Check sheet for the drawn part. Datum: minimum x, y, z corner. Units: mm. Coordinates: 2 decimals unless noted, no trailing zeros. Loops run counter-clockwise (first coordinate to the right, second up) from the corner with the lowest first, then second, coordinate; pieces in that order, holes last.
Q1. Material ranges on probe 1 along X at (y, z) = (16.5, 1.2); probe 2 along Y at (x, z) = (29, 1.2), recorded low to high.
Q2. Sectioned sample at A-A (y = 13.25). Enter the section's corners in (x, z), then the cut area to 3 significant figures.
Q3. Sectioned sample at B-B (z = 0.7). Enter the section's corners in (x, y).
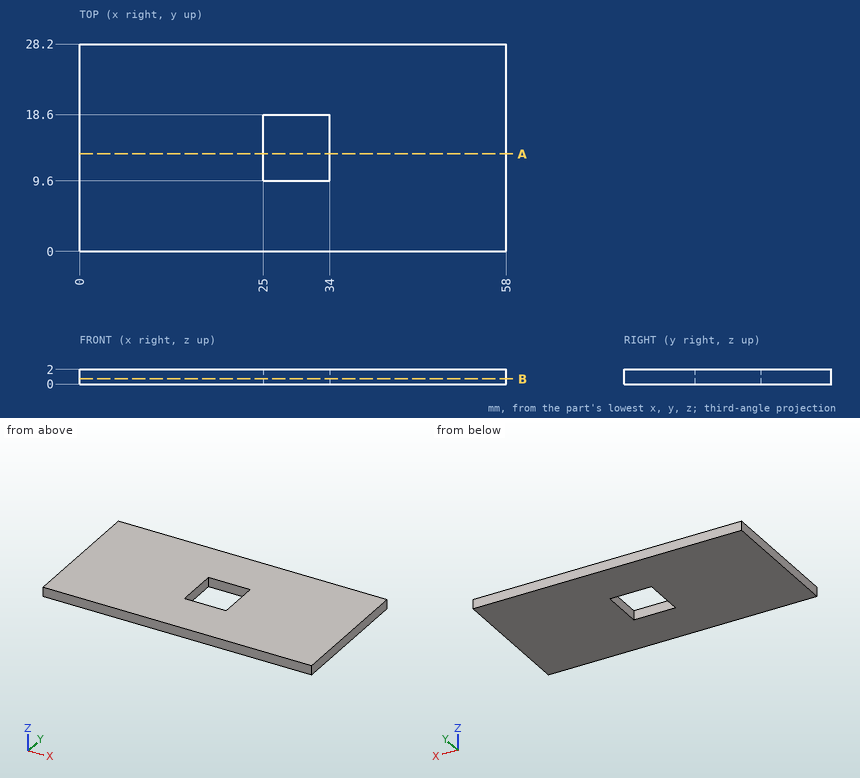
Geometry check:
1. probe 1: x = 0 to 25, 34 to 58
1. probe 2: y = 0 to 9.6, 18.6 to 28.2
2. outline: (0, 0) - (25, 0) - (25, 2) - (0, 2) - close; (34, 0) - (58, 0) - (58, 2) - (34, 2) - close
2. area: 98.0 mm2
3. outline: (0, 0) - (58, 0) - (58, 28.2) - (0, 28.2) - close; hole (25, 9.6) - (34, 9.6) - (34, 18.6) - (25, 18.6) - close
